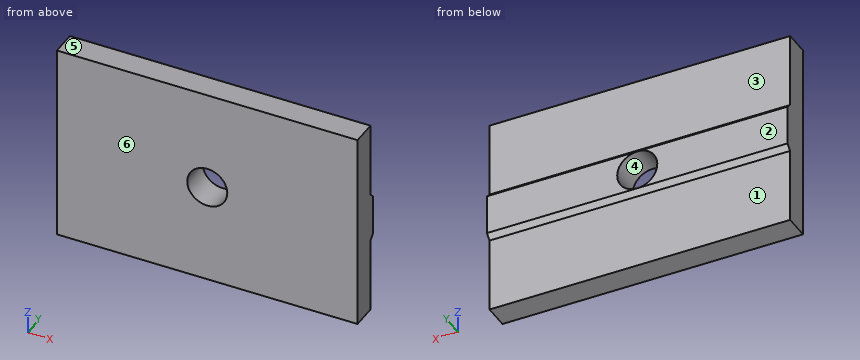
from build123d import *

# Parameters (mm, degrees)
SZKIC1_W                        = 60
SZKIC1_H                        = 40
DODANIE_WYCI_GNI_CIE1_DEPTH     = 5
SZKIC2_W                        = 60
SZKIC2_H                        = 10
DODANIE_WYCI_GNI_CIE2_DEPTH     = 6
SFAZOWANIE1_SIZE                = 1
WYTNIJ_WYCI_GNI_CIE1_DEPTH      = 37.551333765
WYTNIJ_WYCI_GNI_CIE1_DEPTH_BACK = 37.551333765
SZKIC3_R                        = 4


with BuildPart() as part:
    # Szkic1 → Dodanie-wyciągnięcie1 (new body)
    with BuildSketch(Plane(origin=(0, 0, 0), x_dir=(1, 0, 0), z_dir=(0, 1, 0))):
        Rectangle(SZKIC1_W, SZKIC1_H)
    extrude(amount=DODANIE_WYCI_GNI_CIE1_DEPTH)

    # Szkic2 → Dodanie-wyciągnięcie2 (add)
    with BuildSketch(Plane(origin=(0, 0, 0), x_dir=(1, 0, 0), z_dir=(0, 1, 0))):
        Rectangle(SZKIC2_W, SZKIC2_H)
    extrude(amount=DODANIE_WYCI_GNI_CIE2_DEPTH)

    # Sfazowanie1
    sfazowanie1_edges = [part.edges().sort_by_distance(p)[0] for p in [
        (0, 6, -5),
        (0, 6, 5),
    ]]
    chamfer(sfazowanie1_edges, length=SFAZOWANIE1_SIZE - 0.0001)  # a hair under: the kernel refuses the full size

    # Szkic3 → Wytnij-wyciągnięcie1 (cut, two sides: drawn at the far end of the back side and taken through both)
    with BuildSketch(Plane(origin=(0, 0, 0), x_dir=(1, 0, 0), z_dir=(0, 1, 0)).offset(-WYTNIJ_WYCI_GNI_CIE1_DEPTH_BACK)):
        with Locations(Location((0, 0, 0), (0, 0, 270))):
            Circle(SZKIC3_R)
    extrude(amount=WYTNIJ_WYCI_GNI_CIE1_DEPTH + WYTNIJ_WYCI_GNI_CIE1_DEPTH_BACK, mode=Mode.SUBTRACT)


solid = part.part
The model under review builds one solid part; all positions refer to its coordinate system, in mm. Face numbers are marked on the shaded views. A direction names the side the tool comes from. Give positions to 0.01 mm unless a question says otherwise; leave off trailing zeros. Loops run counter-clockwise (first coordinate to the right, second up) from the corner with the lowest first, then second, coordinate; pieces in that order, holes last. Notation, with made-up numbers: (76.5, 37.5) -> (110.5, 37.5) arc R13 ccw to (110.5, 47.5) -> close; hole circle Ø2 at (45.25, 2). An arc over 180 degrees is marked (long way). Put each result on its own line as item: value. Start each with the question number.
1. We need section B-B on z = 0. State the section outline as (x, y) points.
2. Mouldability with a two-part tool opening along Z and no side actions: class the marked faces 4, 5 and 6 as released by +Z, released by -Z, zero draft, split by the parting line, or undercut.
3. For the marked faces 1, 2 and 3, list the 3-axis set-ups (+Z, -Z, +X, -X, +Y, -Y) from which the entire face can be reached by the end or side of a thin tool; tool diameter is ignored.
4. Wall thickness on probe 1 along X at (y, z) = (4.1, 0); probe 2 along Z at (x, y) = (0, 2.75); probe 3 along Y at (x, z) = (25.5, -17): over which ranges is each line inside the solid? List them lowest first.
5. We need section D-D on y = 2.25. State the section outline as (x, z) points, then the cut area to 3 significant figures.
6. Clearance check with flat-ended pins moving along their axes: P1, Ø7.5, axis at x = -3.5, z = 11, coming from the +Y side; P2, Ø9, axis at x = 0, z = 0, coming from the +Y side. State where each tip first meets the part, or that it passes through.
Determined:
1. outline: (-30, 0) -> (-4, 0) -> (-4, 6) -> (-30, 6) -> close; (4, 0) -> (30, 0) -> (30, 6) -> (4, 6) -> close
2. face 4: undercut
2. face 5: released by +Z
2. face 6: zero draft
3. face 1: -Z, +X, -X, +Y
3. face 2: +Z, -Z, +X, -X, +Y
3. face 3: +Z, +X, -X, +Y
4. probe 1: -30 to -4, 4 to 30
4. probe 2: -20 to -4, 4 to 20
4. probe 3: 0 to 5
5. outline: (-30, -20) -> (30, -20) -> (30, 20) -> (-30, 20) -> close; hole circle Ø8 at (0, 0)
5. area: 2,350 mm^2
6. P1: y = 5
6. P2: y = 6
